Part print with two shaded views. Sizes in mm from the minimum x, y, z corner. A direction names the side the tool comes from. Coordinates: 2 decimals unless noted, no trailing zeros. Loops run counter-clockwise (first coordinate to the right, second up) from the corner with the lowest first, then second, coordinate; pieces in that order, holes last. Notation, with made-up numbers: (-21.5, -27.75) - (17.5, -27.75) arc R21 cw to (17.5, -19.75) - close; hole circle Ø11 at (-8, 81). An arc over 180 degrees is marked (long way). Answer as CSV lines item,"result".
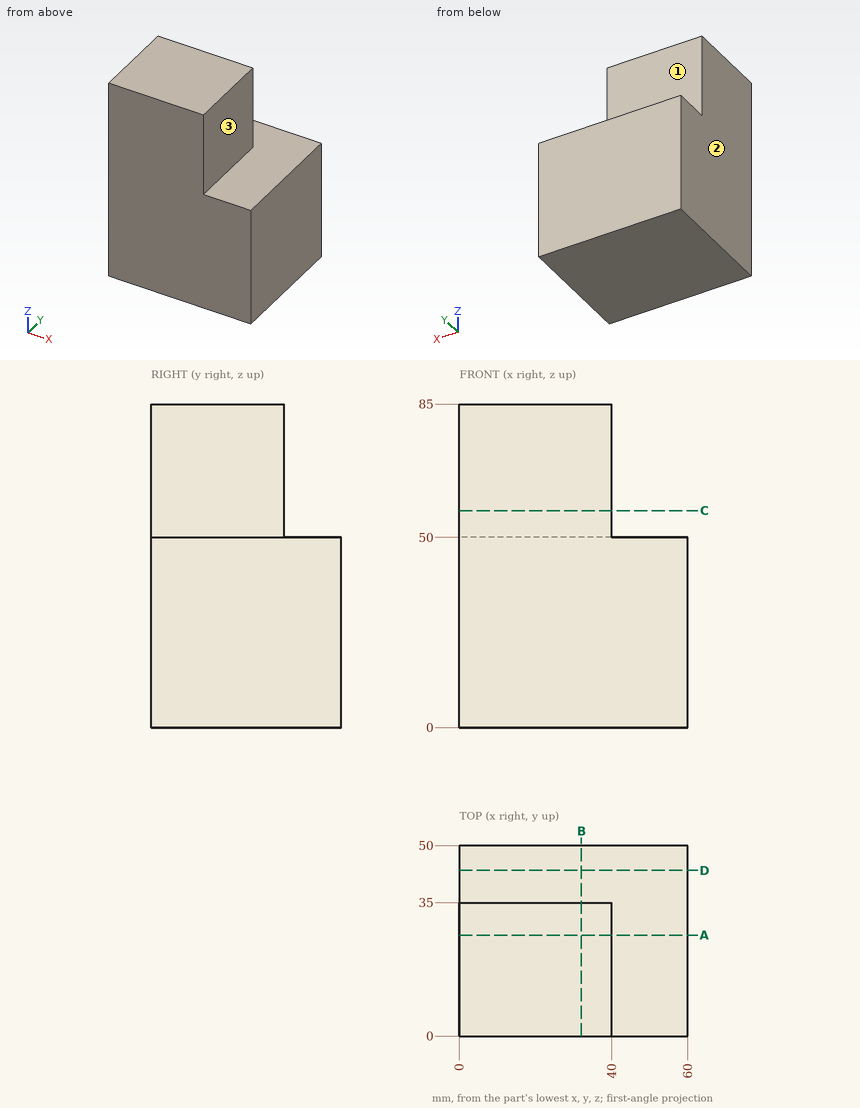
Q1. Saw through at B-B (x = 32). Give the cut face in (y, z), then the cut area to 4 significant figures.
Results:
outline,"(0, 0) - (50, 0) - (50, 50) - (35, 50) - (35, 85) - (0, 85) - close"
area,"3,725 mm^2"
Q2. Which spindle directions (+Z, -Z, +X, -X, +Y, -Y) get a long thin tool onto all of the face, cutting with end or side? Do the marked faces 1, 2 and 3. Say none if no direction does.
Results:
face 1,"+Z, +X, -X, +Y"
face 2,"+Z, -Z, -X, +Y, -Y"
face 3,"+Z, +X, +Y, -Y"
Q3. Saw through at D-D (y = 43.5). Give the cut face in (x, z), then the cut area to 3 significant figures.
Results:
outline,"(0, 0) - (60, 0) - (60, 50) - (0, 50) - close"
area,"3,000 mm^2"
Q4. Wall check: L1, parallel to X at y = 31, z = 64.5; L2, parallel to Y at x = 21.5, z = 71.5; L3, parallel to Z at x = 46, y = 41. Give the ranges that are in metal, low to high.
Results:
L1,"x = 0 to 40"
L2,"y = 0 to 35"
L3,"z = 0 to 50"
Q5. Flat gauge pins, fed straight in: pin 1 (5 mm diameter, centred on x = 23, z = 50.5, fed in from +Y); pin 2 (10 mm diameter, centred on x = 53, y = 26.5, fed in from +Z). Where does each tip first touch, or does it go through?
Results:
pin 1,"stops at y = 50"
pin 2,"stops at z = 50"
Q6. Saw through at A-A (y = 26.5). Give the cut face in (x, z).
Results:
outline,"(0, 0) - (60, 0) - (60, 50) - (40, 50) - (40, 85) - (0, 85) - close"
Q7. Saw through at C-C (z = 57). Give the cut face in (x, y).
Results:
outline,"(0, 0) - (40, 0) - (40, 35) - (0, 35) - close"
